Source: CAD feature listing. Evaluate the final solid. Frame: model axes, mm. Face numbers are marked on the shaded views. A direction names the side the tool comes from. Round coordinates to 2 decimals unless told otherwise and drop trailing zeros. Loops run counter-clockwise (first coordinate to the right, second up) from the corner with the lowest first, then second, coordinate; pieces in that order, holes last. Notation, with made-up numbers: (86.5, 76.5) -> (106.5, 76.5) arc R22 ccw to (106.5, 96.5) -> close; hole circle Ø5 at (-7, 8.25). An arc over 180 degrees is marked (long way). Put each result on its own line as item: value. Start each with the question number.
1. Contact query for flat-ended pins moving along their axis: pin 1 (6 mm diameter, centred on x = -82, z = -11.5, fed in from -Y); pin 2 (1.5 mm diameter, centred on x = -74, z = -7.5, fed in from +Y); pin 3 (6.5 mm diameter, centred on x = -89, y = 291.5, fed in from +Z). Output: stop coordinate, or through.
2. Cut plane C-C (z = 4). Return the cut outline in (x, y), then the cut area to 3 significant figures.
3. Cut plane B-B (y = 56). Return the cut outline in (x, z), then the cut area to 3 significant figures.
4. Material intervals for L1, parallel to Y at x = -90, z = -48.75; L2, parallel to Z at x = 162.5, y = -31; L3, parallel to Y at x = -66.5, z = 46.5, sorted ascending.
5. Set-up query: the marked faces 5 and 6. Return all of +Z, -Z, +X, -X, +Y, -Y with unobstructed straight access to the full face (end or side cutting, diameter ignored); none if empty.
6. Cut plane D-D (x = -24.5). Return the cut outline in (y, z).
7. Cut plane A-A (z = -27). Return the cut outline in (x, y).
8. Draft query along Y for the marked faces 1, 2, 3 and 4. Return one class per face: pulls with the +Y half, pulls with the -Y half, needs draft (parallel to the pull), parting line crosses it, or undercut.
```python
from build123d import *

# Parameters (mm, degrees)
SKETCH1_W           = 330
SKETCH1_H           = 120
BOSS_EXTRUDE1_DEPTH = 120
SKETCH2_W           = 100
SKETCH2_H           = 100
CUT_EXTRUDE1_DEPTH  = 357.230262611
CUT_EXTRUDE2_REACH  = 214.662
SKETCH5_W           = 330
SKETCH5_H           = 80
SKETCH6_W           = 40
SKETCH6_H           = 20
BOSS_EXTRUDE2_DEPTH = 180
SKETCH9_R           = 4
BOSS_EXTRUDE3_DEPTH = 25
SKETCH11_W          = 20
SKETCH11_H          = 120
EXTRUDE_THIN1_DEPTH = 120
CUT_EXTRUDE3_REACH  = 359.526
SKETCH12_W          = 30
SKETCH12_H          = 100
EXTRUDE_THIN2_DEPTH = 50
BOSS_EXTRUDE5_DEPTH = 20
FILLET1_R           = 10
SKETCH9_4_R         = 11
CUT_EXTRUDE4_DEPTH  = 367.367302034
SKETCH17_W          = 50
SKETCH17_H          = 20
BOSS_EXTRUDE6_DEPTH = 180
FILLET6_R           = 10


with BuildPart() as part:
    # Sketch1 → Boss-Extrude1 (new body)
    with BuildSketch(Plane(origin=(0, 0, 0), x_dir=(1, 0, 0), z_dir=(0, 1, 0))):
        Rectangle(SKETCH1_W, SKETCH1_H)
    extrude(amount=BOSS_EXTRUDE1_DEPTH)

    # Sketch2 → Cut-Extrude1 (cut, through all)
    with BuildSketch(Plane(origin=(165, 0, 0), x_dir=(0, 0, -1), z_dir=(1, 0, 0))):
        with Locations((0, 60)):
            Rectangle(SKETCH2_W, SKETCH2_H)
    extrude(amount=-CUT_EXTRUDE1_DEPTH, mode=Mode.SUBTRACT)

    # Sketch5 → Cut-Extrude2 (cut, up to next)
    with BuildSketch(Plane(origin=(0, 120, 0), x_dir=(1, 0, 0), z_dir=(0, 1, 0)), mode=Mode.PRIVATE) as cut_extrude2_sk1:
        Rectangle(SKETCH5_W, SKETCH5_H)
    cut_extrude2_tool1 = extrude(cut_extrude2_sk1.sketch, amount=-CUT_EXTRUDE2_REACH, mode=Mode.PRIVATE) & part.part
    add(cut_extrude2_tool1.solids().sort_by_distance((0, 120, 0))[0], mode=Mode.SUBTRACT)

    # Sketch6 → Boss-Extrude2 (add)
    with BuildSketch(Plane(origin=(0, 120, 0), x_dir=(1, 0, 0), z_dir=(0, 1, 0))):
        with Locations((-95, 50)):
            Rectangle(SKETCH6_W, SKETCH6_H)
    extrude(amount=BOSS_EXTRUDE2_DEPTH)

    # Sketch9 → Boss-Extrude3 (add)
    with BuildSketch(Plane.XY.offset(-40)):
        with Locations(Location((-90, 290, 0), (0, 0, 180))):
            Circle(SKETCH9_R)
    extrude(amount=BOSS_EXTRUDE3_DEPTH)

    # Sketch11 → Extrude-Thin1 (add, through all)
    with BuildSketch(Plane(origin=(0, 120, 0), x_dir=(1, 0, 0), z_dir=(0, 1, 0))):
        with Locations((175, 0)):
            Rectangle(SKETCH11_W, SKETCH11_H)
    extrude(amount=-EXTRUDE_THIN1_DEPTH)

    # Sketch12 → Cut-Extrude3 (cut, up to next)
    with BuildSketch(Plane.XZ, mode=Mode.PRIVATE) as cut_extrude3_sk1:
        with Locations((150, 0)):
            Rectangle(SKETCH12_W, SKETCH12_H)
    cut_extrude3_tool1 = extrude(cut_extrude3_sk1.sketch, amount=-CUT_EXTRUDE3_REACH, mode=Mode.PRIVATE) & part.part
    add(cut_extrude3_tool1.solids().sort_by_distance((150, 0, 0))[0], mode=Mode.SUBTRACT)

    # Sketch14 → Extrude-Thin2 (add)
    with BuildSketch(Plane.XZ):
        Polygon((-165, -60), (185, -60), (185, 60), (-165, 60), (-165, 50), (175, 50), (175, -50), (-165, -50), align=None)
    extrude(amount=EXTRUDE_THIN2_DEPTH)

    # Sketch16 → Boss-Extrude5 (add, through all)
    with BuildSketch(Plane.XY.offset(-40)):
        Polygon((-75, 300), (75, 120), (-75, 120), align=None)
    extrude(amount=-BOSS_EXTRUDE5_DEPTH)

    # Fillet1
    fillet1_edges = [part.edges().sort_by_distance(p)[0] for p in [
        (-75, 300, -50),
    ]]
    fillet(fillet1_edges, radius=FILLET1_R)

    # Sketch9<4> → Cut-Extrude4 (cut, through all)
    with BuildSketch(Plane.XY.offset(-40)):
        with Locations((-90, 190)):
            Circle(SKETCH9_4_R)
    extrude(amount=-CUT_EXTRUDE4_DEPTH, mode=Mode.SUBTRACT)

    # Sketch17 → Boss-Extrude6 (add, through all)
    with BuildSketch(Plane(origin=(0, 120, 0), x_dir=(1, 0, 0), z_dir=(0, 1, 0))):
        with Locations((-140, 50)):
            Rectangle(SKETCH17_W, SKETCH17_H)
    extrude(amount=BOSS_EXTRUDE6_DEPTH)

    # Fillet6
    fillet6_edges = [part.edges().sort_by_distance(p)[0] for p in [
        (-165, 120, 50),
        (-165, 300, -50),
    ]]
    fillet(fillet6_edges, radius=FILLET6_R)


solid = part.part
```
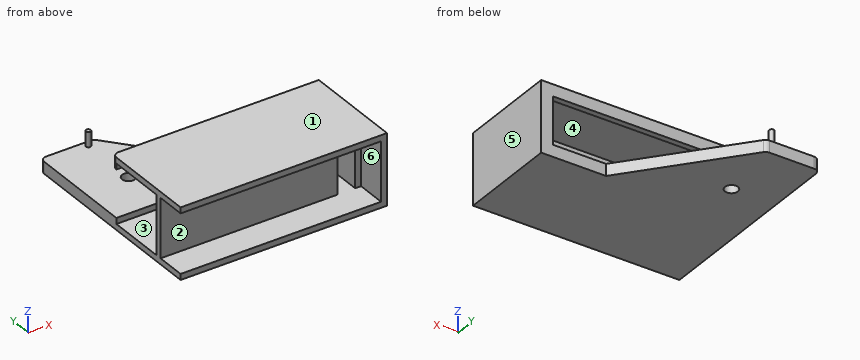
Solution:
1. pin 1: stops at y = 0
1. pin 2: stops at y = 10
1. pin 3: stops at z = -15
2. outline: (-165, 0) -> (135, 0) -> (135, 10) -> (-165, 10) -> close; (165, 0) -> (175, 0) -> (175, -50) -> (185, -50) -> (185, 120) -> (165, 120) -> close
2. area: 5,900 mm^2
3. outline: (-165, -60) -> (185, -60) -> (185, 60) -> (-165, 60) -> (-165, 50) -> (165, 50) -> (165, -50) -> (-165, -50) -> close
3. area: 9,000 mm^2
4. L1: y = 0 to 10, 110 to 179, 201 to 300
4. L2: z = -60 to -50, 50 to 60
4. L3: y = 0 to 10, 110 to 120
5. face 5: +Z, -Z, +X, +Y, -Y
5. face 6: -X, -Y
6. outline: (-50, -60) -> (239.4, -60) -> (239.4, -40) -> (110, -40) -> (110, -50) -> (10, -50) -> (10, 50) -> (110, 50) -> (110, 40) -> (120, 40) -> (120, 60) -> (-50, 60) -> (-50, 50) -> (0, 50) -> (0, -50) -> (-50, -50) -> close
7. outline: (-165, 0) -> (135, 0) -> (135, 10) -> (-165, 10) -> close; circle Ø8 at (-90, 290); (165, 0) -> (175, 0) -> (175, -50) -> (185, -50) -> (185, 120) -> (165, 120) -> close
8. face 1: needs draft
8. face 2: pulls with the -Y half
8. face 3: undercut
8. face 4: undercut
